Build history of the part. All positions in model axes, mm. A direction names the side the tool comes from. Round coordinates to 2 decimals unless told otherwise and drop trailing zeros. Write each loop counter-clockwise with the first axis right and the second up, starting at its lowest first coordinate (ties: lowest second). Pieces come first, ordered by that corner, then holes. Notation, with made-up numbers: (72, 5) - (81, 5) arc R34 cw to (81, 38) - close; hole circle Ø4 at (88, -36.5). An arc over 180 degrees is marked (long way). One line per question, with ' | ' between items.
from build123d import *

# Parameters (mm, degrees)
SKETCH3_W           = 192
SKETCH3_H           = 135
BOSS_EXTRUDE1_DEPTH = 5.7
CUT_EXTRUDE1_DEPTH  = 6
SKETCH11_R          = 1
CUT_EXTRUDE2_DEPTH  = 33


with BuildPart() as part:
    # Sketch3 → Boss-Extrude1 (new body)
    with BuildSketch(Plane(origin=(0, 0, 0), x_dir=(1, 0, 0), z_dir=(0, 1, 0))):
        with Locations((90, 53.5)):
            Rectangle(SKETCH3_W, SKETCH3_H)
    extrude(amount=BOSS_EXTRUDE1_DEPTH)

    # Sketch4 → Cut-Extrude1 (cut)
    with BuildSketch(Plane(origin=(0, 0, 0), x_dir=(1, 0, 0), z_dir=(0, 1, 0))):
        Polygon((-5.7, 121.001666615), (-5.7, 94), (0, 94), (0, 67), (-5.7, 67), (-5.7, 40), (0, 40), (0, 13), (-5.7, 13), (-5.7, -17), (-9.7, -17), (-9.7, 121.001666615), align=None)
        Polygon((189.7, 121.001666615), (185.7, 121.001666615), (185.7, 94), (180, 94), (180, 67), (185.7, 67), (185.7, 40), (180, 40), (180, 13), (185.7, 13), (185.7, -17), (189.7, -17), align=None)
    extrude(amount=CUT_EXTRUDE1_DEPTH, mode=Mode.SUBTRACT)

    # Sketch11 → Cut-Extrude2 (cut)
    with BuildSketch(Plane(origin=(0, 0, 0), x_dir=(1, 0, 0), z_dir=(0, 1, 0))):
        with Locations((99, 53.5)):
            Circle(SKETCH11_R)
        with Locations((154.2, 53.5)):
            Circle(SKETCH11_R)
    extrude(amount=CUT_EXTRUDE2_DEPTH, mode=Mode.SUBTRACT)


solid = part.part
Q1. Saw through at B-B, the plane z = -31. List the corners of the cut face in (x, y), then the cut area to 3 significant figures.
Found:
outline: (0, 0) - (180, 0) - (180, 5.7) - (0, 5.7) - close | area: 1,030 mm^2
Q2. Which spindle directions (+Z, -Z, +X, -X, +Y, -Y) get a long thin tool onto all of the face, cutting with end or side? Do faces 1 (the flat face through (-3, 3, -40)), 2 (the flat face through (185.7, 3, -108)), 3 (the flat face through (183, 3, -40)). Say none if no direction does.
Found:
face 1: -X, +Y, -Y | face 2: +Z, -Z, +X, +Y, -Y | face 3: +X, +Y, -Y
Q3. Drill centre lines: L1, parallel to X at y = 4.55, z = -53.5; L2, parallel to Z at x = 154.2, y = 2.1; L3, parallel to X at y = 3, z = -24.5. Where is each one in solid material? Low to high. Write a range as from..to.
Found:
L1: -5.7..98, 100..153.2, 155.2..185.7 | L2: -121..-54.5, -52.5..14 | L3: 0..180
Q4. Drop flat-ended pins along their axis: pin 1 (1.5 mm diameter, centred on y = 4.5, z = -74.5, fed in from -X); pin 2 (2.5 mm diameter, centred on x = 99, z = -53.5, fed in from +Y); pin 3 (1.7 mm diameter, centred on y = 2.5, z = -84, fed in from +X); pin 4 (1.8 mm diameter, centred on x = 154.2, z = -53.5, fed in from -Y) (3 decimals). Give the stop position or say it passes through.
Found:
pin 1: x = 0 | pin 2: y = 5.7 | pin 3: x = 180 | pin 4: through
Q5. Saw through at A-A, the plane y = 4.45. List the corners of the cut face in (x, z), then the cut area to 3 significant figures.
Found:
outline: (-5.7, -121) - (185.7, -121) - (185.7, -94) - (180, -94) - (180, -67) - (185.7, -67) - (185.7, -40) - (180, -40) - (180, -13) - (185.7, -13) - (185.7, 14) - (-5.7, 14) - (-5.7, -13) - (0, -13) - (0, -40) - (-5.7, -40) - (-5.7, -67) - (0, -67) - (0, -94) - (-5.7, -94) - close; hole circle Ø2 at (99, -53.5); hole circle Ø2 at (154.2, -53.5) | area: 25,200 mm^2
